```python
from build123d import *

# Parameters (mm, degrees)
F0_W     = 25
F0_H     = 15
F0_R     = 1
F0_R_2   = 2
F0_R_3   = 0.5
F1_DEPTH = 5
F2_DEPTH = 3


with BuildPart() as f1:
    # F0 (on Front) → F1 (new body)
    with BuildSketch(Plane.XZ):
        Rectangle(F0_W, F0_H)
        with Locations((-10.5, -5.5)):
            Circle(F0_R, mode=Mode.SUBTRACT)
        with Locations((10.5, -5.5)):
            Circle(F0_R, mode=Mode.SUBTRACT)
        with Locations((-7, 0)):
            Circle(F0_R_2, mode=Mode.SUBTRACT)
        with Locations((-10.5, 5.5)):
            Circle(F0_R, mode=Mode.SUBTRACT)
        with BuildLine():
            ThreePointArc((6, 0), (4, -2), (2, 0))
            ThreePointArc((2, 0), (4, 2), (6, 0))
        make_face(mode=Mode.SUBTRACT)
        with Locations((10.5, 5.5)):
            Circle(F0_R, mode=Mode.SUBTRACT)
        with Locations((-7, 0)):
            Circle(F0_R_2)
        with Locations((-7, 0)):
            Circle(F0_R_3, mode=Mode.SUBTRACT)
        with BuildLine():
            ThreePointArc((6, 0), (4, 2), (2, 0))
            ThreePointArc((2, 0), (4, -2), (6, 0))
        make_face()
        with BuildLine():
            ThreePointArc((4.5, 0), (4, -0.5), (3.5, 0))
            ThreePointArc((3.5, 0), (4, 0.5), (4.5, 0))
        make_face(mode=Mode.SUBTRACT)
        with Locations((-7, 0)):
            Circle(F0_R_3)
        with BuildLine():
            ThreePointArc((4.5, 0), (4, 0.5), (3.5, 0))
            ThreePointArc((3.5, 0), (4, -0.5), (4.5, 0))
        make_face()
    extrude(amount=F1_DEPTH)

    # F0 (on Front) → F2 (cut)
    with BuildSketch(Plane.XZ):
        with Locations((-7, 0)):
            Circle(F0_R_2)
        with Locations((-7, 0)):
            Circle(F0_R_3, mode=Mode.SUBTRACT)
        with BuildLine():
            ThreePointArc((6, 0), (4, 2), (2, 0))
            ThreePointArc((2, 0), (4, -2), (6, 0))
        make_face()
        with BuildLine():
            ThreePointArc((4.5, 0), (4, -0.5), (3.5, 0))
            ThreePointArc((3.5, 0), (4, 0.5), (4.5, 0))
        make_face(mode=Mode.SUBTRACT)
        with BuildLine():
            ThreePointArc((4.5, 0), (4, 0.5), (3.5, 0))
            ThreePointArc((3.5, 0), (4, -0.5), (4.5, 0))
        make_face()
        with Locations((-7, 0)):
            Circle(F0_R_3)
    extrude(amount=F2_DEPTH, mode=Mode.SUBTRACT)


solid = f1.part
```
Geometry check sheet. Reference: the model listing, model coordinates, mm. A direction names the side the tool comes from. Coordinates: 2 decimals unless noted, no trailing zeros. Write each loop counter-clockwise with the first axis right and the second up, starting at its lowest first coordinate (ties: lowest second). Pieces come first, ordered by that corner, then holes. Notation, with made-up numbers: M -11,-11.75 L 41,-11.75 A10 ccw 41,-3.75 Z; hole C 29.5,79 d5. An arc over 180 degrees is marked long. One line per item, written item: value. Start each with the question number.
(1) Sectioned sample at C-C, the plane y = -0.4. Enter the section's corners in (x, z), and give its area (3 significant figures).
(2) Release check for a two-part mould opening along Z. For faces 3 (the face through (4, -3, 0)), 4 (the face through (12.5, -2, 0)), 5 (the face through (-11.237, -2.465, -4.824)), 6 (the face through (0, -2, -7.5)) record: released by +Z, released by -Z, zero draft, split by the parting line, or undercut.
(3) Sectioned sample at A-A, the plane x = -10.5. Enter the section's corners in (y, z).
(4) Scan lines: line 1 along Z through (x, y) = (10.5, -3.7); line 2 along X through (y, z) = (-1.8, -5); line 3 along X through (y, z) = (-0.8, -1.25). Record each from-to range of solid material in increasing order. Write a range as [from, to].
(5) Depth check by flat-ended pin: pin 1 (1.8 mm diameter, centred on x = 10.5, z = -5.5, fed in from -Y); pin 2 (1.2 mm diameter, centred on x = 4.5, z = -0.5, fed in from +Y). Enter the tip coordinate at first touch or a pass-through.
(6) Sectioned sample at D-D, the plane y = -3.75. Enter the section's corners in (x, z).
(7) Sectioned sample at B-B, the plane z = -5.5. Enter the section's corners in (x, y), and give its area (3 significant figures).
(8) Tool access check on faces 1 (the face through (0, -5, 0)), 2 (the face through (-7, -3, 0)). Record the directions out of +Z, -Z, +X, -X, +Y, -Y that give a thin tool (end or side, any length) a straight path to the whole face; none if there is none.
Filled sheet:
1. outline: M -12.5,-7.5 L 12.5,-7.5 L 12.5,7.5 L -12.5,7.5 Z; hole C -10.5,-5.5 d2; hole C -10.5,5.5 d2; hole C -7,0 d4; hole C 4,0 d4; hole C 10.5,-5.5 d2; hole C 10.5,5.5 d2
1. area: 337 mm²
2. face 3: undercut
2. face 4: zero draft
2. face 5: undercut
2. face 6: released by -Z
3. outline: M -5,-7.5 L 0,-7.5 L 0,-6.5 L -5,-6.5 Z; M -5,-4.5 L 0,-4.5 L 0,4.5 L -5,4.5 Z; M -5,6.5 L 0,6.5 L 0,7.5 L -5,7.5 Z
4. line 1: [-7.5, -6.5], [-4.5, 4.5], [6.5, 7.5]
4. line 2: [-12.5, -11.37], [-9.63, 9.63], [11.37, 12.5]
4. line 3: [-12.5, -8.56], [-5.44, 2.44], [5.56, 12.5]
5. pin 1: through
5. pin 2: y = -3
6. outline: M -12.5,-7.5 L 12.5,-7.5 L 12.5,7.5 L -12.5,7.5 Z; hole C -10.5,-5.5 d2; hole C -10.5,5.5 d2; hole C 10.5,-5.5 d2; hole C 10.5,5.5 d2
7. outline: M -12.5,-5 L -11.5,-5 L -11.5,0 L -12.5,0 Z; M -9.5,-5 L 9.5,-5 L 9.5,0 L -9.5,0 Z; M 11.5,-5 L 12.5,-5 L 12.5,0 L 11.5,0 Z
7. area: 105 mm²
8. face 1: +Z, -Z, +X, -X, -Y
8. face 2: +Y
